Autodesk Fusion 360 part; units mm, degrees
sketch "草图1" plane through (0, 0, 0) normal (0, 0, 1) x (1, 0, 0) in component "support"
  line L0 (40.3306, 33.6594) -> (40.3306, -61.561)
  line L1 (40.3306, -61.561) -> (-18.6734, -36.5899)
  line L2 (-18.6734, -36.5899) -> (-18.6734, 5.8967)
  line L3 (-18.6734, 5.8967) -> (24.5506, 5.8967)
  line L4 (24.5506, 5.8967) -> (24.5506, 28.4577)
  line L5 (24.5506, 28.4577) -> (40.3306, 33.6594)
  line L6 (35.2823, 8.3501) -> (35.2823, 23.9544)
  arc A0 (35.2823, 23.9544) -> (29.8253, 23.9544) centre (32.5538, 23.9544) ccw
  line L7 (29.8253, 23.9544) -> (29.8253, 8.3501)
  arc A1 (29.8253, 8.3501) -> (35.2823, 8.3501) centre (32.5538, 8.3501) ccw
  line L8 (32.5538, 5.6216) -> (32.5538, 26.6829) construction
  line L9 (-13.4908, -5.8932) -> (34.7153, -6.5796)
  line L10 (34.7153, -6.5796) -> (34.7153, 0.2419)
  line L11 (-18.6734, -11.6226) -> (24.884, -12.2428)
  line L12 (24.884, -12.2428) -> (22.3355, -19.0792)
  line L13 (-7.9409, -29.2052) -> (-18.6734, -29.2052)
  line L14 (35, -20.4957) -> (35, -51.1893)
  line L15 (-13.4908, 0.2419) -> (-13.4908, -5.8932)
  line L16 (34.7153, 0.2419) -> (-13.4908, 0.2419)
  line L17 (35, -51.1893) -> (10.8843, -40.9833)
  line L18 (10.8843, -40.9833) -> (35, -20.4957)
  line L19 (12.9862, -29.3446) -> (22.3355, -19.0792)
  line L20 (12.9862, -29.3446) -> (7.5042, -29.3446)
  arc A2 (-7.9409, -29.2052) -> (7.5042, -29.3446) centre (-0.2208, -29.5486) ccw
extrude "拉伸4" add sketch "草图1" along normal blind 20 contours L0 L1 L2 L3 L4 L5 L11 L12 L13 L19 L20 A2 in component "support"
fillet "圆角22" radius 2 1 edges at (10.8843, -40.9833, 10) in component "support"
fillet "圆角23" radius 2 1 edges at (35, -51.1893, 10) in component "support"
fillet "圆角24" radius 2 1 edges at (35, -20.4957, 10) in component "support"
fillet "圆角25" radius 5 1 edges at (40.3306, -61.561, 10) in component "support"
fillet "圆角26" radius 5 1 edges at (40.3306, 33.6594, 10) in component "support"
fillet "圆角27" radius 5 1 edges at (24.5506, 28.4577, 10) in component "support"
fillet "圆角28" radius 2 1 edges at (24.5506, 5.8967, 10) in component "support"
fillet "圆角29" radius 5 2 edges at (-18.6734, 5.8967, 10) (-18.6734, -11.6226, 10) in component "support"
fillet "圆角30" radius 2 1 edges at (-18.6734, -29.2052, 10) in component "support"
fillet "圆角31" radius 2 1 edges at (-18.6734, -36.5899, 10) in component "support"
fillet "圆角32" radius 2 1 edges at (34.7153, 0.2419, 10) in component "support"
fillet "圆角33" radius 2 1 edges at (34.7153, -6.5796, 10) in component "support"
fillet "圆角34" radius 2 1 edges at (-13.4908, -5.8932, 10) in component "support"
fillet "圆角35" radius 2 1 edges at (-13.4908, 0.2419, 10) in component "support"
fillet "圆角36" radius 0.5 1 edges at (24.884, -12.2428, 10) in component "support"
fillet "圆角37" radius 1 1 edges at (22.3355, -19.0792, 10) in component "support"
fillet "圆角38" radius 2 1 edges at (12.9862, -29.3446, 10) in component "support"
fillet "圆角39" radius 3 1 edges at (-7.9409, -29.2052, 10) in component "support"
fillet "圆角40" radius 3 1 edges at (7.5042, -29.3446, 10) in component "support"
component "support" placed x (1, 0, 0) y (0, 1, 0) z (0, 0, 1) at (0, 0, 0)
Read the model definition and answer for the solid it produces. Units are mm, in the model's axes. A direction names the side the tool comes from. Round coordinates to 2 decimals unless told otherwise and drop trailing zeros. Loops run counter-clockwise (first coordinate to the right, second up) from the corner with the lowest first, then second, coordinate; pieces in that order, holes last.
Q1. Each of these flat-tipped pins is pushed along its axis until it touches: pin 1 (4 mm diameter, centred on x = -7.5, z = 17, fed in from +Y); pin 2 (1 mm diameter, centred on y = -45.5, z = 9.5, fed in from -X); pin 3 (3 mm diameter, centred on y = 8.5, z = 3, fed in from -X). Where does it stop, or does it pass through?
Q2. Determine the mould class of faces 4 (the face through (8.32, -48.014, 9.86)), 5 (the face through (11, 0.242, 10)), 6 (the face through (-14, -29.205, 10)), 7 (the face through (40.331, -13, 10)) for opening direction X: released by +X, released by -X, zero draft, split by the parting line, or undercut.
Q3. Section A-A on y = 15.5 is taken. Write down the section's boundary in (x, z), and give its area (3 significant figures).
Q4. Section B-B on x = 3 is taken. Write down the section's boundary in (y, z), and give its area (3 significant figures).
Q5. Section C-C on y = -34 is taken. Write down the section's boundary in (x, z).
Q6. Which of the six approach directions +Z, -Z, +X, -X, +Y, -Y give full straight-line access (tool end or side, diameter ignored) to faces 1 (the face through (24.551, 16, 10)), 2 (the face through (11, -29.345, 10)), 3 (the face through (24, -17, 0))?
Q7. Consider probe 1 along Y at (x, z) = (12.5, 15.5); probe 2 along X at (y, z) = (8, 16.25); probe 3 along X at (y, z) = (-34, 7). Determine where each line is inside the solid, lowest interval first.
Q8. Section D-D on z = 2 is taken. Give the number of separate pieces and of enclosed holes in the cut face, and give its area (3 significant figures).
Output:
1. pin 1: stops at y = 5.9
1. pin 2: stops at x = 1.2
1. pin 3: stops at x = 24.34
2. face 4: released by -X
2. face 5: undercut
2. face 6: zero draft
2. face 7: released by +X
3. outline: (24.55, 0) - (29.83, 0) - (29.83, 20) - (24.55, 20) - close; (35.28, 0) - (40.33, 0) - (40.33, 20) - (35.28, 20) - close
3. area: 206 mm2
4. outline: (-45.76, 0) - (-36.57, 0) - (-36.57, 20) - (-45.76, 20) - close; (-11.93, 0) - (-6.13, 0) - (-6.13, 20) - (-11.93, 20) - close; (0.24, 0) - (5.9, 0) - (5.9, 20) - (0.24, 20) - close
4. area: 413 mm2
5. outline: (-18.67, 0) - (-6.54, 0) - (-6.54, 20) - (-18.67, 20) - close; (6.1, 0) - (19.1, 0) - (19.1, 20) - (6.1, 20) - close; (35, 0) - (40.33, 0) - (40.33, 20) - (35, 20) - close
6. face 1: +Z, -Z, -X, +Y
6. face 2: +Z, -Z
6. face 3: -Z, +X, -X, +Y, -Y
7. probe 1: y = -49.78 to -29.3, -12.07 to -6.26, 0.24 to 5.9
7. probe 2: x = 24.55 to 29.85, 35.26 to 40.33
7. probe 3: x = -18.67 to -6.54, 6.1 to 19.1, 35 to 40.33
8. separate pieces: 1
8. enclosed holes: 3
8. area: 2,050 mm2
